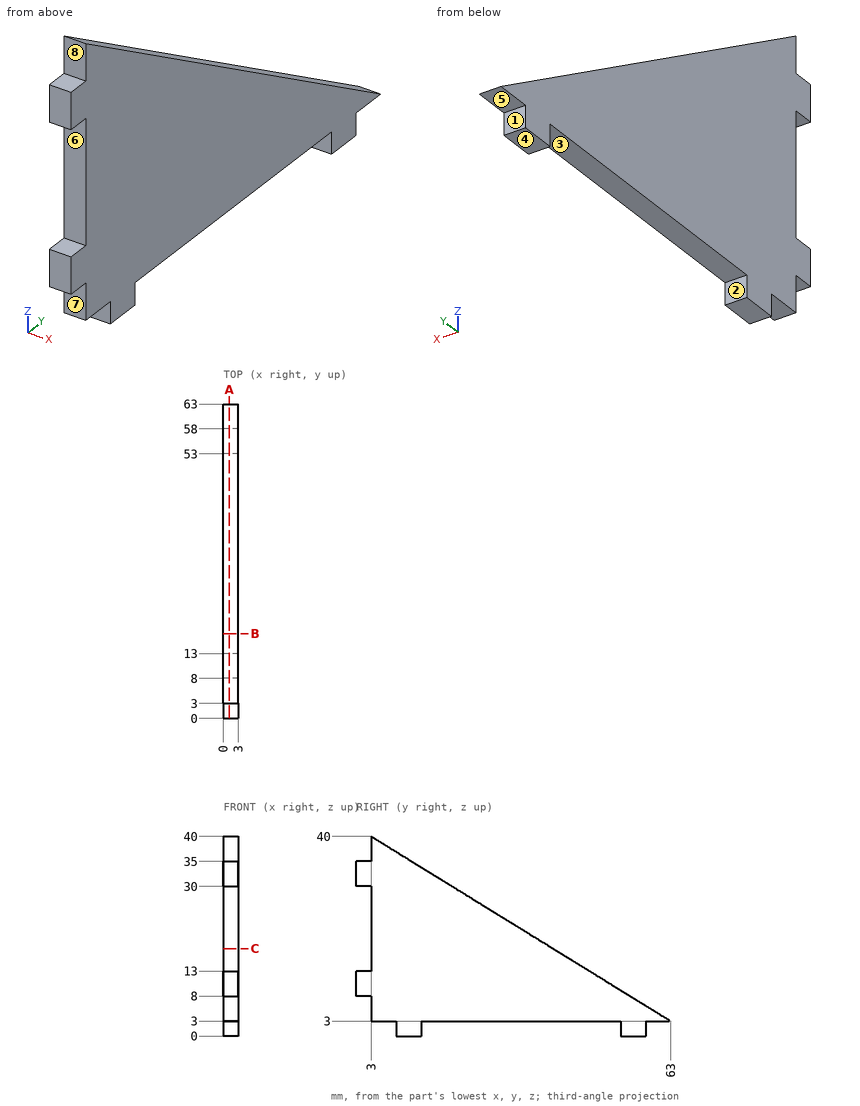
Drawing for the job (mm, zero at the part's lowest x, y, z). A direction names the side the tool comes from. Round coordinates to 2 decimals unless told otherwise and drop trailing zeros. Loops run counter-clockwise (first coordinate to the right, second up) from the corner with the lowest first, then second, coordinate; pieces in that order, holes last. Notation, with made-up numbers: M -39.75,46 L -19.75,46 A28 cw -19.75,70 Z; hole C -34,-11 d3. An arc over 180 degrees is marked long. Use a Markdown table: item, result. Add a question column.
(1) Flat gauge pins, fed straight in: pin 1 (1.5 mm diameter, centred on x = 2, y = 2, fed in from +Z); pin 2 (1 mm diameter, centred on x = 1.5, y = 33.5, fed in from +Z); pin 3 (1 mm diameter, centred on x = 1, z = 8, fed in from -Y); pin 4 (1.5 mm diameter, centred on x = 0.5, z = 32, fed in from +Y). Where does each tip first touch, or does it go through?
(2) Cut at B-B (y = 17). Give the cut face in (x, z), and give its area (3 significant figures).
(3) Pull direction Y, two halves, no side cores. Call the marked faces 1, 2, 3 and 4: +Y half, -Y half, draft (parallel to the pull), parting line (faces both ways), or undercut.
(4) Which spindle directions (+Z, -Z, +X, -X, +Y, -Y) get a long thin tool onto all of the face, cutting with end or side? Do the marked faces 5, 6, 7 and 8. Say none if no direction does.
(5) Cut at A-A (x = 1.2). Give the cut face in (y, z).
(6) Cut at C-C (z = 17.5). Give the cut face in (x, y), and give its area (3 significant figures).
(7) Drill centre lines: line 1 (Z direction, x = 2.25, y = 24); line 2 (Y direction, x = 0.95, z = 27); line 3 (Z direction, x = 0.55, y = 45). Where is each one in solid material? Low to high.
Geometry says:
| question | item | result |
|---|---|---|
| 1 | pin 1 | stops at z = 35 |
| 1 | pin 2 | stops at z = 21.5 |
| 1 | pin 3 | stops at y = 0 |
| 1 | pin 4 | stops at y = 17.19 |
| 2 | outline | M 0,3 L 3,3 L 3,31.37 L 0,31.37 Z |
| 2 | area | 85.1 mm² |
| 3 | face 1 | +Y half |
| 3 | face 2 | undercut |
| 3 | face 3 | undercut |
| 3 | face 4 | draft |
| 4 | face 5 | -Z, +X, -X, +Y |
| 4 | face 6 | +X, -X, -Y |
| 4 | face 7 | -Z, +X, -X, -Y |
| 4 | face 8 | +Z, +X, -X, -Y |
| 5 | outline | M 0,8 L 3,8 L 3,3 L 8,3 L 8,0 L 13,0 L 13,3 L 53,3 L 53,0 L 58,0 L 58,3 L 63,3 L 3,40 L 3,35 L 0,35 L 0,30 L 3,30 L 3,13 L 0,13 Z |
| 6 | outline | M 0,3 L 3,3 L 3,39.49 L 0,39.49 Z |
| 6 | area | 109 mm² |
| 7 | line 1 | z = 3 to 27.05 |
| 7 | line 2 | y = 3 to 24.08 |
| 7 | line 3 | z = 3 to 14.1 |
